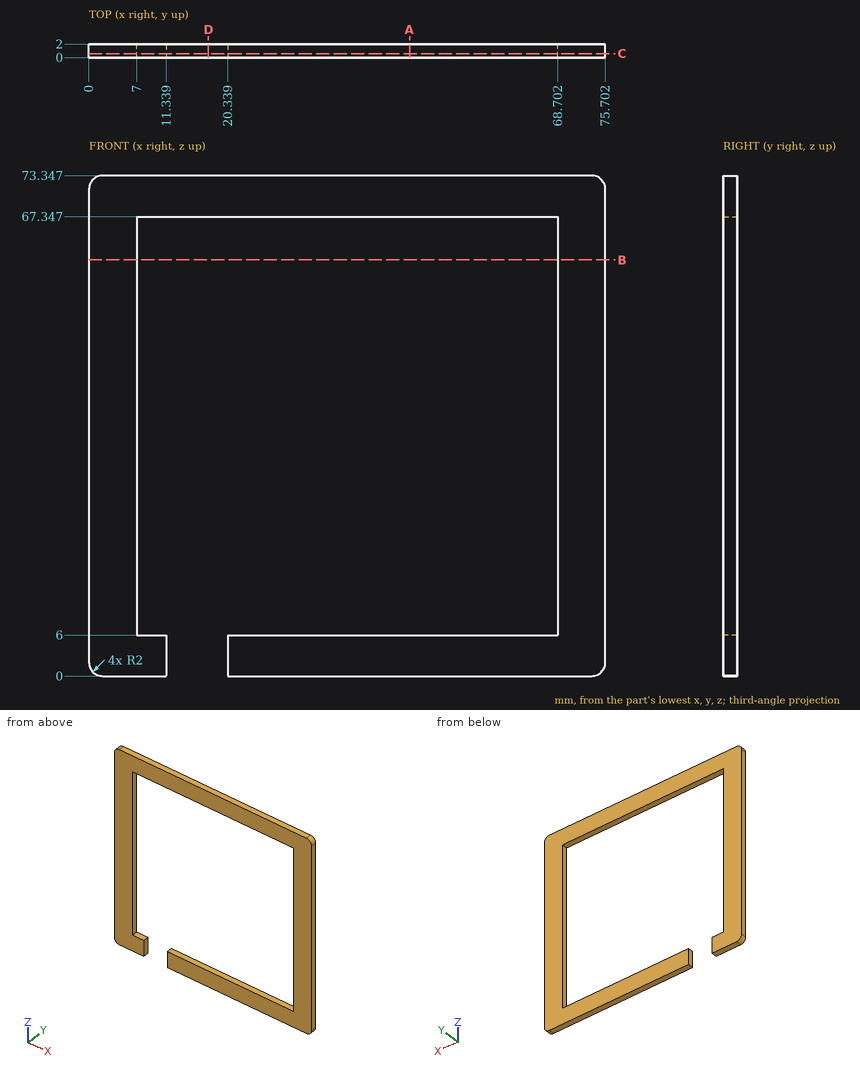
Here's the drawing with two shaded views (mm, measured from the low corner). I have some questions. Give positions to 0.01 mm unless a question says otherwise; leave off trailing zeros. Order: outer loops, then holes, each group sorted by start corner. A loop starts at its lowest first (then second) coordinate and runs counter-clockwise, first axis right, second up. Notation, with made-up numbers: (11.25, 0) -> (26.25, 0) arc R13 ccw to (26.25, 19) -> close; hole circle Ø5 at (6, 78.5). An arc over 180 degrees is marked (long way). Use a Markdown table: item, result. Add a question column.
Item 1: I need wall thicknesses on line 1 (Z direction, x = 55, y = 0.7); line 2 (X direction, y = 0.9, z = 27.5); line 3 (Z direction, x = 15, y = 1.9). Which ranges of each line are inside material? Lowest first, please.
Item 2: Will this pin go through, and if not, where does the flat tip stop? pin 1 (1 mm diameter, centred on y = 1.5, z = 2, fed in from -X).
Item 3: Imagine slicing it at A-A on x = 47. Please give me the cut outline in (y, z).
Item 4: Imagine slicing it at B-B on z = 61. Please give me the cut outline in (x, y).
Item 5: Imagine slicing it at D-D on x = 17.5. Please give me the cut outline in (y, z).
Item 6: Imagine slicing it at C-C on y = 0.6. Please give me the cut outline in (x, z), plus the area to 3 significant figures.
Data:
| question | item | result |
|---|---|---|
| 1 | line 1 | z = 0 to 6, 67.35 to 73.35 |
| 1 | line 2 | x = 0 to 7, 68.7 to 75.7 |
| 1 | line 3 | z = 67.35 to 73.35 |
| 2 | pin 1 | stops at x = 0 |
| 3 | outline | (0, 0) -> (2, 0) -> (2, 6) -> (0, 6) -> close; (0, 67.35) -> (2, 67.35) -> (2, 73.35) -> (0, 73.35) -> close |
| 4 | outline | (0, 0) -> (7, 0) -> (7, 2) -> (0, 2) -> close; (68.7, 0) -> (75.7, 0) -> (75.7, 2) -> (68.7, 2) -> close |
| 5 | outline | (0, 67.35) -> (2, 67.35) -> (2, 73.35) -> (0, 73.35) -> close |
| 6 | outline | (0, 2) arc R2 ccw to (2, 0) -> (11.34, 0) -> (11.34, 6) -> (7, 6) -> (7, 67.35) -> (68.7, 67.35) -> (68.7, 6) -> (20.34, 6) -> (20.34, 0) -> (73.7, 0) arc R2 ccw to (75.7, 2) -> (75.7, 71.35) arc R2 ccw to (73.7, 73.35) -> (2, 73.35) arc R2 ccw to (0, 71.35) -> close |
| 6 | area | 1,710 mm² |
